Study the drawing (mm; zero at the part's minimum x, y, z) and answer. Give positions to 0.01 mm unless a question says otherwise; leave off trailing zeros. Order: outer loops, then holes, each group sorted by start corner. A loop starts at its lowest first (then second) coordinate and runs counter-clockwise, first axis right, second up. Notation, with made-up numbers: (44, 18) -> (56, 18) arc R18 cw to (56, 47) -> close; hole circle Ø6 at (70.25, 27). An arc over 180 degrees is marked (long way). One line per question, with ' | ' between items. Start each with the question number.
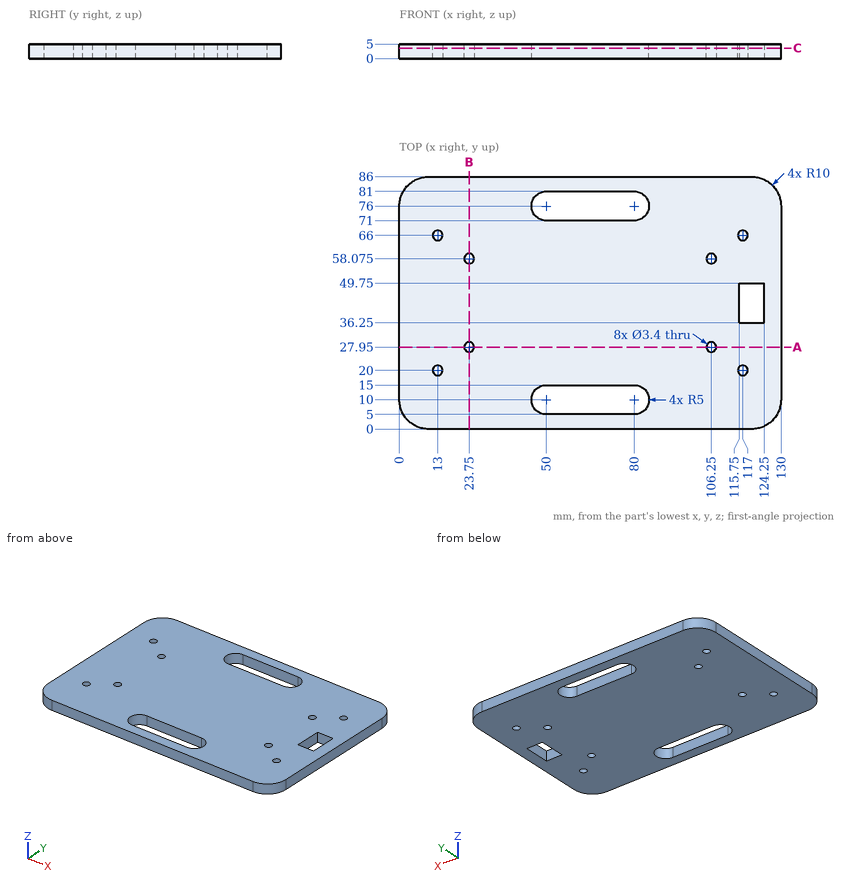
Q1. A cutting plane is placed at A-A, the plane y = 27.95. Determine the outline of the cut face in (x, z), then the cut area to 3 significant figures.
Q2. A cutting plane is placed at C-C, the plane z = 3.6. Give the number of separate pieces and of enclosed holes in the cut face, then the cut area to 3 significant figures.
Q3. Find the intervals of material crossed by line 1 (Y direction, x = 117, z = 2.2); line 2 (Y direction, x = 106.25, z = 3.7) (3 decimals); line 3 (Y direction, x = 68, z = 0.45), in increasing order.
Q4. A cutting plane is placed at B-B, the plane x = 23.75. Determine the outline of the cut face in (y, z) (3 decimals), then the cut area to 3 significant figures.
Geometry results:
1) outline: (0, 0) -> (22.05, 0) -> (22.05, 5) -> (0, 5) -> close; (25.45, 0) -> (104.55, 0) -> (104.55, 5) -> (25.45, 5) -> close; (107.95, 0) -> (130, 0) -> (130, 5) -> (107.95, 5) -> close | area: 616 mm²
2) separate pieces: 1 | enclosed holes: 11 | area: 10,100 mm²
3) line 1: 0 to 18.3, 21.7 to 36.25, 49.75 to 64.3, 67.7 to 86 | line 2: 0 to 26.25, 29.65 to 56.375, 59.775 to 86 | line 3: 0 to 5, 15 to 71, 81 to 86
4) outline: (0, 0) -> (26.25, 0) -> (26.25, 5) -> (0, 5) -> close; (29.65, 0) -> (56.375, 0) -> (56.375, 5) -> (29.65, 5) -> close; (59.775, 0) -> (86, 0) -> (86, 5) -> (59.775, 5) -> close | area: 396 mm²
